from build123d import *

# Parameters (mm, degrees)
BOSS_EXTRU_1_DEPTH      = 45
ESQUISSE2_R             = 8
ENL_V_MAT_EXTRU_1_DEPTH = 50
ESQUISSE3_R             = 2
ENL_V_MAT_EXTRU_2_DEPTH = 50
ESQUISSE4_R             = 1.8
ESQUISSE4_R_2           = 7
ENL_V_MAT_EXTRU_3_DEPTH = 5
BOSS_EXTRU_2_DEPTH      = 60
BOSS_EXTRU_3_DEPTH      = 45
ESQUISSE11_W            = 8
ESQUISSE11_H            = 8
ESQUISSE11_R            = 2.3
ESQUISSE11_R_2          = 2.268048231
BOSS_EXTRU_6_DEPTH      = 6
ESQUISSE12_W            = 40
ESQUISSE12_H            = 12
ESQUISSE12_W_2          = 45
ENL_V_MAT_EXTRU_5_DEPTH = 50
ESQUISSE13_W            = 5
ESQUISSE13_H            = 12
ENL_V_MAT_EXTRU_6_DEPTH = 20
ESQUISSE25_R            = 13.4
ENL_V_MAT_EXTRU_8_DEPTH = 2


with BuildPart() as part:
    # Esquisse1 → Boss.-Extru.1 (new body)
    with BuildSketch(Plane(origin=(0, 0, 0), x_dir=(1, 0, 0), z_dir=(0, 1, 0))):
        Polygon((-15, 0), (17, 0), (17, 50), (12, 50), (12, 6), (-10, 6), (-10, 103), (-15, 103), align=None)
    extrude(amount=BOSS_EXTRU_1_DEPTH)

    # Esquisse2 → Enl_v. mat.-Extru.1 (cut)
    with BuildSketch(Plane(origin=(17, 0, 0), x_dir=(0, 0, -1), z_dir=(1, 0, 0))):
        with Locations((30, 18)):
            Circle(ESQUISSE2_R)
    extrude(amount=-ENL_V_MAT_EXTRU_1_DEPTH, mode=Mode.SUBTRACT)

    # Esquisse3 → Enl_v. mat.-Extru.2 (cut)
    with BuildSketch(Plane.ZY.offset(15)):
        with BuildLine():
            Line((-52, 27), (-52, 37))
            ThreePointArc((-52, 37), (-54, 35), (-56, 37))
            Line((-56, 37), (-56, 27))
            ThreePointArc((-56, 27), (-54, 29), (-52, 27))
        make_face()
        with Locations((-54, 37)):
            Circle(ESQUISSE3_R)
        with Locations((-54, 27)):
            Circle(ESQUISSE3_R)
    extrude(amount=-ENL_V_MAT_EXTRU_2_DEPTH, mode=Mode.SUBTRACT)

    # Esquisse4 → Enl_v. mat.-Extru.3 (cut)
    with BuildSketch(Plane(origin=(-10, 0, 0), x_dir=(0, 0, -1), z_dir=(1, 0, 0))):
        with Locations((85, 8)):
            Circle(ESQUISSE4_R)
        with Locations((95, 18)):
            Circle(ESQUISSE4_R)
        with Locations((75, 18)):
            Circle(ESQUISSE4_R)
        with Locations((85, 28)):
            Circle(ESQUISSE4_R)
        with Locations((85, 18)):
            Circle(ESQUISSE4_R_2)
    extrude(amount=-ENL_V_MAT_EXTRU_3_DEPTH, mode=Mode.SUBTRACT)

    # Esquisse4_4 → Boss.-Extru.2 (add)
    with BuildSketch(Plane(origin=(-10, 0, 0), x_dir=(0, 0, -1), z_dir=(1, 0, 0))):
        Polygon((94, 0), (103, 0), (103, 8.072261083), (94, 8.072261083), (94, 4.036130542), align=None)
        Polygon((67, 0), (76, 0), (76, 4), (76, 8.072261083), (67, 8.072261083), align=None)
        Polygon((76, 0), (94, 0), (94, 4.036130542), (76, 4), align=None)
    extrude(amount=-BOSS_EXTRU_2_DEPTH)

    # Esquisse6 → Boss.-Extru.3 (add)
    with BuildSketch(Plane.XZ):
        Polygon((-5, -6), (-10, -6), (-10, -16), (-5, -11), (7, -11), (12, -16), (12, -6), (7, -6), align=None)
    extrude(amount=-BOSS_EXTRU_3_DEPTH)

    # Esquisse11 → Boss.-Extru.6 (add)
    # profile 1 of 7: a face of its own
    with BuildSketch(Plane.XZ):
        with Locations((13, 4)):
            Rectangle(ESQUISSE11_W, ESQUISSE11_H)
        with Locations(Location((13, 4, 0), (0, 0, 270))):
            Circle(ESQUISSE11_R, mode=Mode.SUBTRACT)
    # profile 2 of 7: a face of its own
    with BuildSketch(Plane.XZ):
        Polygon((17, -58), (17, -50), (12, -50), (12, -46), (9, -46), (9, -58), align=None)
        with Locations(Location((13, -54, 0), (0, 0, 270))):
            Circle(ESQUISSE11_R, mode=Mode.SUBTRACT)
    # profile 3 of 7: a face of its own
    with BuildSketch(Plane.XZ):
        with Locations((-11, 4)):
            Rectangle(ESQUISSE11_W, ESQUISSE11_H)
        with Locations(Location((-11, 4, 0), (0, 0, 270))):
            Circle(ESQUISSE11_R_2, mode=Mode.SUBTRACT)
    # profile 4 of 7: a face of its own
    with BuildSketch(Plane.XZ):
        with Locations((-66, -63)):
            Rectangle(ESQUISSE11_W, ESQUISSE11_H)
        with Locations(Location((-66, -63, 0), (0, 0, 270))):
            Circle(ESQUISSE11_R, mode=Mode.SUBTRACT)
    # profile 5 of 7: a face of its own
    with BuildSketch(Plane.XZ):
        with Locations((-66, -107)):
            Rectangle(ESQUISSE11_W, ESQUISSE11_H)
        with Locations(Location((-66, -107, 0), (0, 0, 270))):
            Circle(ESQUISSE11_R, mode=Mode.SUBTRACT)
    # profile 6 of 7: a face of its own
    with BuildSketch(Plane.XZ):
        with Locations((-14, -107)):
            Rectangle(ESQUISSE11_W, ESQUISSE11_H)
        with Locations(Location((-14, -107, 0), (0, 0, 270))):
            Circle(ESQUISSE11_R, mode=Mode.SUBTRACT)
    # profile 7 of 7: a face of its own
    with BuildSketch(Plane.XZ):
        with Locations((-27, -107)):
            Rectangle(ESQUISSE11_W, ESQUISSE11_H)
        with Locations(Location((-27, -107, 0), (0, 0, 270))):
            Circle(ESQUISSE11_R, mode=Mode.SUBTRACT)
    extrude(amount=-BOSS_EXTRU_6_DEPTH)

    # Esquisse12 → Enl_v. mat.-Extru.5 (cut)
    with BuildSketch(Plane.ZY.offset(15)):
        with Locations((-83, 39)):
            Rectangle(ESQUISSE12_W, ESQUISSE12_H)
        with Locations((-22.5, 39)):
            Rectangle(ESQUISSE12_W_2, ESQUISSE12_H)
    extrude(amount=-ENL_V_MAT_EXTRU_5_DEPTH, mode=Mode.SUBTRACT)

    # Esquisse13 → Enl_v. mat.-Extru.6 (cut)
    with BuildSketch(Plane(origin=(17, 0, 0), x_dir=(0, 0, -1), z_dir=(1, 0, 0))):
        with Locations((47.5, 39)):
            Rectangle(ESQUISSE13_W, ESQUISSE13_H)
    extrude(amount=-ENL_V_MAT_EXTRU_6_DEPTH, mode=Mode.SUBTRACT)

    # Esquisse25 → Enl_v. mat.-Extru.8 (cut)
    with BuildSketch(Plane.ZY.offset(15)):
        with Locations((-85, 18)):
            Circle(ESQUISSE25_R)
    extrude(amount=-ENL_V_MAT_EXTRU_8_DEPTH, mode=Mode.SUBTRACT)


solid = part.part
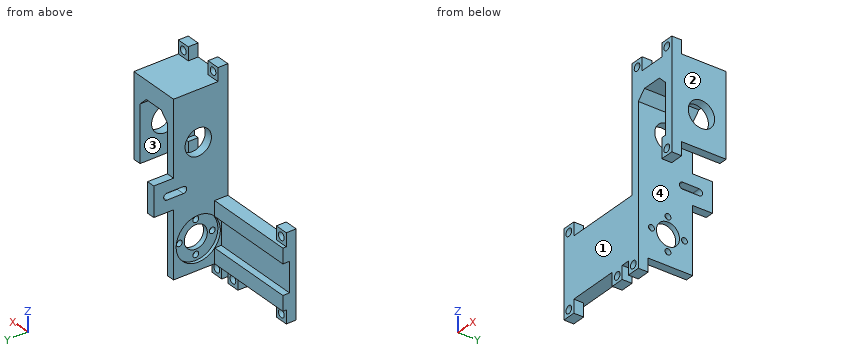
Could you check a few things on this model? Use its own coordinates, in mm. Face numbers are marked on the shaded views. Round coordinates to 2 decimals unless told otherwise and drop trailing zeros. Order: outer loops, then holes, each group sorted by start corner. A loop starts at its lowest first (then second) coordinate and runs counter-clockwise, first axis right, second up.
Q1. Imagine slicing it at B-B, the plane z = -107. List the corners of the cut face in (x, y) for me, then the cut area to 3 significant figures.
Geometry says:
outline: (-70, 0) - (-68.3, 0) - (-68.3, 6) - (-70, 6) - close; (-63.7, 0) - (-62, 0) - (-62, 6) - (-63.7, 6) - close; (-31, 0) - (-29.3, 0) - (-29.3, 6) - (-31, 6) - close; (-24.7, 0) - (-23, 0) - (-23, 6) - (-24.7, 6) - close; (-18, 0) - (-16.3, 0) - (-16.3, 6) - (-18, 6) - close; (-11.7, 0) - (-10, 0) - (-10, 6) - (-11.7, 6) - close
area: 61.2 mm2
Q2. Please list where these lines run through material, in increasing order: probe 1 along X at (y, z) = (2, -107); probe 2 along X at (y, z) = (25, -35.5); probe 3 along X at (y, z) = (4.2, -63).
Geometry says:
probe 1: x = -70 to -68.3, -63.7 to -62, -31 to -29.3, -24.7 to -23, -18 to -16.3, -11.7 to -10
probe 2: x = -15 to -10, 12 to 17
probe 3: x = -70 to -68.3, -63.7 to -62, -15 to -10
Q3. I'm going to push flat-ended pins straight in: P1, Ø10, axis at x = -34, z = -99, coming from the +Y side; P2, Ø6, axis at y = 30.5, z = -98.5, coming from the -X side; P3, Ø3, axis at x = 14, y = 4.5, coming from the -Z side. Where does each tip first touch, or does it pass through?
Geometry says:
P1: stops at y = 8.07
P2: stops at x = -15
P3: stops at z = -58
Q4. Thinking about a two-plate mould opening in X: for the marked faces 1, 2, 3 and 4, which applies, released by +X, released by -X, zero draft, split by the parting line, or undercut?
Geometry says:
face 1: zero draft
face 2: released by +X
face 3: undercut
face 4: undercut
Q5. Imagine slicing it at C-C, the plane y = 18. State how many separate pieces and enclosed holes the cut face has, then the cut area to 3 significant figures.
Geometry says:
separate pieces: 6
enclosed holes: 0
area: 755 mm2
Q6. Imagine slicing it at A-A, the plane x = -66. List the corners of the cut face in (y, z) for me, then the cut area to 3 significant figures.
Geometry says:
outline: (0, -111) - (6, -111) - (6, -109.3) - (0, -109.3) - close; (0, -104.7) - (6, -104.7) - (6, -103) - (8.07, -103) - (8.07, -94) - (4.04, -94) - (4, -76) - (8.07, -76) - (8.07, -67) - (6, -67) - (6, -65.3) - (0, -65.3) - close; (0, -60.7) - (6, -60.7) - (6, -59) - (0, -59) - close
area: 258 mm2
Q7. Imagine slicing it at D-D, the plane z = -17.5. List the corners of the cut face in (x, y) for me.
Geometry says:
outline: (-15, 0) - (-10, 0) - (-10, 33) - (-15, 33) - close; (12, 0) - (17, 0) - (17, 33) - (12, 33) - close
